from build123d import *

# Parameters (mm, degrees)
F0_R     = 1.25
F0_R_2   = 4.5
F1_DEPTH = 5
F0_W     = 11.7265549134
F0_H     = 7.858
F0_R_3   = 1.6
F2_DEPTH = 2.5
F0_W_2   = 7.858
F0_H_2   = 11.7265549134
F3_DEPTH = 5
F4_DEPTH = 2.5
F5_DEPTH = 1
F6_R     = 175
F8_DEPTH = 25


# Not quite as in the source:
# - a feature names something its author has since deleted; it is built from what else it names


with BuildPart() as f1:
    # F0 (on Top) → F1 (new body)
    with BuildSketch(Plane.XY):
        with BuildLine():
            Line((-10.2734450866, -3.929), (-22, -3.929))
            Line((-22, -3.929), (-22, -4.058874503))
            ThreePointArc((-22, -4.058874503), (-23.2179274798, -10.1818094209), (-26.686291501, -15.372583002))
            Line((-26.686291501, -15.372583002), (-78.0019548635, -66.6882463645))
            ThreePointArc((-78.0019548635, -66.6882463645), (-91.9238815543, -91.9238815543), (-66.6882463645, -78.0019548635))
            Line((-66.6882463645, -78.0019548635), (-15.372583002, -26.686291501))
            ThreePointArc((-15.372583002, -26.686291501), (-10.1818094209, -23.2179274798), (-4.058874503, -22))
            Line((-4.058874503, -22), (-3.929, -22))
            Line((-3.929, -22), (-3.929, -10.2734450866))
            Line((-3.929, -10.2734450866), (-5.9698516934, -8.2325933932))
            Line((-5.9698516934, -8.2325933932), (-18.3937554159, -20.6564971157))
            Line((-18.3937554159, -20.6564971157), (-15.6360389693, -23.4142135624))
            ThreePointArc((-15.6360389693, -23.4142135624), (-15.3431457505, -24.1213203436), (-15.6360389693, -24.8284271247))
            Line((-15.6360389693, -24.8284271247), (-68.3544854934, -77.5468736488))
            ThreePointArc((-68.3544854934, -77.5468736488), (-90.8632213825, -90.8632213825), (-77.5468736488, -68.3544854934))
            Line((-77.5468736488, -68.3544854934), (-24.8284271247, -15.6360389693))
            ThreePointArc((-24.8284271247, -15.6360389693), (-24.1213203436, -15.3431457505), (-23.4142135624, -15.6360389693))
            Line((-23.4142135624, -15.6360389693), (-20.6564971157, -18.3937554159))
            Line((-20.6564971157, -18.3937554159), (-8.2325933932, -5.9698516934))
            Line((-8.2325933932, -5.9698516934), (-10.2734450866, -3.929))
        make_face()
        with BuildLine():
            Line((-18.3937554159, -20.6564971157), (-20.6564971157, -18.3937554159))
            Line((-20.6564971157, -18.3937554159), (-23.4142135624, -15.6360389693))
            ThreePointArc((-23.4142135624, -15.6360389693), (-24.1213203436, -15.3431457505), (-24.8284271247, -15.6360389693))
            Line((-24.8284271247, -15.6360389693), (-77.5468736488, -68.3544854934))
            ThreePointArc((-77.5468736488, -68.3544854934), (-90.8632213825, -90.8632213825), (-68.3544854934, -77.5468736488))
            Line((-68.3544854934, -77.5468736488), (-15.6360389693, -24.8284271247))
            ThreePointArc((-15.6360389693, -24.8284271247), (-15.3431457505, -24.1213203436), (-15.6360389693, -23.4142135624))
            Line((-15.6360389693, -23.4142135624), (-18.3937554159, -20.6564971157))
        make_face()
        with Locations((-81.3172798365, -90.8172798365)):
            Circle(F0_R, mode=Mode.SUBTRACT)
        with Locations((-89.3172798365, -81.3172798365)):
            Circle(F0_R, mode=Mode.SUBTRACT)
        with Locations((-81.3172798365, -81.3172798365)):
            Circle(F0_R_2, mode=Mode.SUBTRACT)
        with Locations((-73.3172798365, -81.3172798365)):
            Circle(F0_R, mode=Mode.SUBTRACT)
        with Locations((-81.3172798365, -71.8172798365)):
            Circle(F0_R, mode=Mode.SUBTRACT)
    extrude(amount=F1_DEPTH)

    # F0 (on Top) → F2 (join)
    with BuildSketch(Plane.XY):
        with Locations((-16.1367225433, 0)):
            Rectangle(F0_W, F0_H)
        with Locations((-15, 0)):
            Circle(F0_R_3, mode=Mode.SUBTRACT)
    extrude(amount=F2_DEPTH)

    # F0 (on Top) → F3 (join)
    with BuildSketch(Plane.XY):
        with Locations((0, -16.1367225433)):
            Rectangle(F0_W_2, F0_H_2)
        with Locations((0, -15)):
            Circle(F0_R_3, mode=Mode.SUBTRACT)
    extrude(amount=F3_DEPTH)

    # F0 (on Top) → F4 (cut)
    with BuildSketch(Plane.XY):
        with Locations((0, -16.1367225433)):
            Rectangle(F0_W_2, F0_H_2)
        with Locations((0, -15)):
            Circle(F0_R_3, mode=Mode.SUBTRACT)
    extrude(amount=F4_DEPTH, mode=Mode.SUBTRACT)

    # F0 (on Top) → F5 (cut)
    with BuildSketch(Plane.XY):
        with BuildLine():
            Line((-18.3937554159, -20.6564971157), (-20.6564971157, -18.3937554159))
            Line((-20.6564971157, -18.3937554159), (-23.4142135624, -15.6360389693))
            ThreePointArc((-23.4142135624, -15.6360389693), (-24.1213203436, -15.3431457505), (-24.8284271247, -15.6360389693))
            Line((-24.8284271247, -15.6360389693), (-77.5468736488, -68.3544854934))
            ThreePointArc((-77.5468736488, -68.3544854934), (-90.8632213825, -90.8632213825), (-68.3544854934, -77.5468736488))
            Line((-68.3544854934, -77.5468736488), (-15.6360389693, -24.8284271247))
            ThreePointArc((-15.6360389693, -24.8284271247), (-15.3431457505, -24.1213203436), (-15.6360389693, -23.4142135624))
            Line((-15.6360389693, -23.4142135624), (-18.3937554159, -20.6564971157))
        make_face()
        with Locations((-81.3172798365, -90.8172798365)):
            Circle(F0_R, mode=Mode.SUBTRACT)
        with Locations((-89.3172798365, -81.3172798365)):
            Circle(F0_R, mode=Mode.SUBTRACT)
        with Locations((-81.3172798365, -81.3172798365)):
            Circle(F0_R_2, mode=Mode.SUBTRACT)
        with Locations((-73.3172798365, -81.3172798365)):
            Circle(F0_R, mode=Mode.SUBTRACT)
        with Locations((-81.3172798365, -71.8172798365)):
            Circle(F0_R, mode=Mode.SUBTRACT)
    extrude(amount=F5_DEPTH, mode=Mode.SUBTRACT)

    # F6
    f6_edges = [f1.edges().sort_by_distance(p)[0] for p in [
        (-66.688246, -78.001955, 2.5),
        (-78.001955, -66.688246, 2.5),
    ]]
    fillet(f6_edges, radius=F6_R)

    # F7 (on face) → F8 (cut)
    with BuildSketch(Plane(origin=(-19.5251262658, -19.5251262658, 0), x_dir=(-0.7071067812, 0.7071067812, 0), z_dir=(0.7071067812, 0.7071067812, 0))):
        Polygon((4.4867513459, 0), (1.6, 5), (1.6, 1), (-1.6, 1), (-1.6, 5), (-4.4867513459, 0), align=None)
    extrude(amount=F8_DEPTH, mode=Mode.SUBTRACT)


solid = f1.part
Here's how the part is built. I have some questions about the finished solid (model axes, mm). A direction names the side the tool comes from. Give positions to 0.01 mm unless a question says otherwise; leave off trailing zeros. Loops run counter-clockwise (first coordinate to the right, second up) from the corner with the lowest first, then second, coordinate; pieces in that order, holes last. Notation, with made-up numbers: (-3, 31) -> (10, 31) arc R21 ccw to (10, 55) -> close; hole circle Ø1 at (-38, 6.25). An arc over 180 degrees is marked (long way). One line per item, written item: value.
Q1. Suppose I cut it at A-A on y = 0. Please give me the cut outline in (x, z).
Answers follow:
outline: (-22, 0) -> (-16.6, 0) -> (-16.6, 2.5) -> (-22, 2.5) -> close; (-13.4, 0) -> (-10.27, 0) -> (-10.27, 2.5) -> (-13.4, 2.5) -> close
Q2. Suppose I cut it at B-B on x = 0. Please give me the cut outline in (y, z).
Answers follow:
outline: (-22, 2.5) -> (-16.6, 2.5) -> (-16.6, 5) -> (-22, 5) -> close; (-13.4, 2.5) -> (-10.27, 2.5) -> (-10.27, 5) -> (-13.4, 5) -> close
Q3. If I drill on line 1 along Y through (x, z) = (0, 3.95); line 2 along Y through (x, z) = (-89, 2.35); line 3 along X through (y, z) = (-9.5, 4.8), over which ranges is the centre line in solid material (lowest first)?
Answers follow:
line 1: -22 to -16.6, -13.4 to -10.27
line 2: -94.2 to -82.53, -80.11 to -68.43
line 3: -22.95 to -11.93, -7.07 to -4.7
Q4. Suppose I cut it at D-D on x = -54. Please give me the cut outline in (y, z), then the cut area to 3 significant figures.
Answers follow:
outline: (-67.25, 0) -> (-63.19, 0) -> (-63.19, 1) -> (-44.81, 1) -> (-44.81, 0) -> (-42.61, 0) -> (-42.61, 5) -> (-67.25, 5) -> close
area: 105 mm^2
Q5. I'm going to push flat-ended pins straight in: pin 1 Ø1 at (y, z) = (-31.5, 2) entering from +X; pin 2 Ø1 at (x, y) = (-55, -59.5) entering from -Z; pin 3 Ø1.2 at (y, z) = (0.5, 0.5) entering from +X. Where does each tip first touch, or does it pass through?
Answers follow:
pin 1: x = -19.69
pin 2: z = 1
pin 3: x = -10.27
Q6. Suppose I cut it at C-C on y = -57.5. Please give me the cut outline in (x, z), then the cut area to 3 significant figures.
Answers follow:
outline: (-71.91, 0) -> (-66.69, 0) -> (-66.69, 1) -> (-48.31, 1) -> (-48.31, 0) -> (-45.85, 0) -> (-45.85, 5) -> (-71.91, 5) -> close
area: 112 mm^2
Q7. We'd pull the mould along X, two halves only. Please class faces 1 (the face through (-3.929, -16, 1)), 2 (the face through (-22, 0, 1)), 3 (the face through (-16.6, 0.07, 1.23)): pulls with the +X half, pulls with the -X half, needs draft (parallel to the pull), parting line crosses it, or undercut.
Answers follow:
face 1: pulls with the +X half
face 2: pulls with the -X half
face 3: undercut
Q8. On a 3-axis mill with a long thin cutter (end or side, diameter ignored), from which of +Z, -Z, +X, -X, +Y, -Y can I reach the whole of each face in a straight line? I mean faces 4 (the face through (-50.82, -41.63, 0.49)), 5 (the face through (-16, -3.929, 4)), 6 (the face through (-10.273, 0, 1)), 7 (the face through (0, -17, 2.5)). Say none if no direction works.
Answers follow:
face 4: -Z
face 5: +Z, +X, -X, +Y
face 6: +Z, -Z, +X, +Y
face 7: -Z, +X, +Y, -Y
